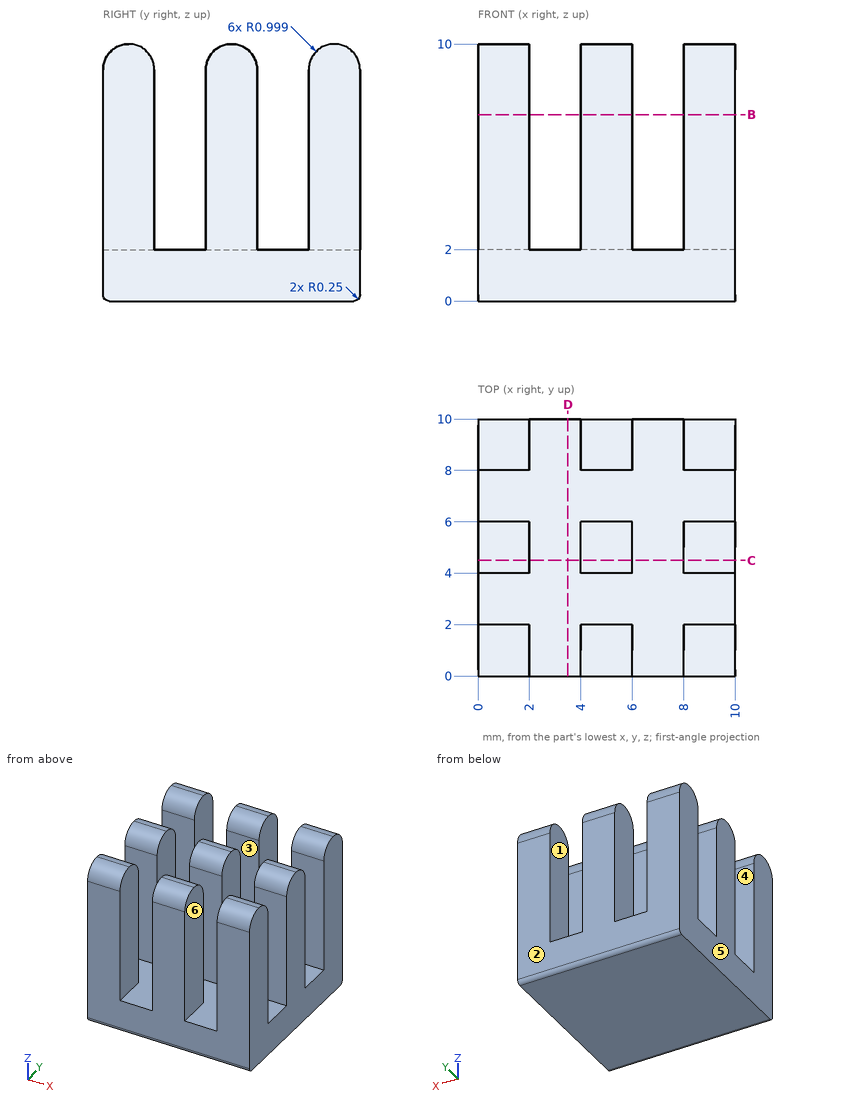
Job drawing, mm, ordinate dimensions from the low corner. One solid piece. A direction names the side the tool comes from. Give positions to 0.01 mm unless a question says otherwise; leave off trailing zeros. Write each loop counter-clockwise with the first axis right and the second up, starting at its lowest first coordinate (ties: lowest second). Pieces come first, ordered by that corner, then holes. Notation, with made-up numbers: (52.25, -23) - (107.25, -23) arc R14 ccw to (107.25, -12) - close; hole circle Ø11 at (9, 12). An arc over 180 degrees is marked (long way). Use one line per item in the form item = value. Start each with the question number.
1. Band-saw the part on D-D on x = 3.5. Write the cut outline in (y, z), plus the area to 3 significant figures.
2. Drop a flat-ended pin along its axis: pin 1 Ø2 at (x, y) = (5.5, 6.5) entering from +Z. Give the stop position or say it passes through.
3. Two-plate mould, pull along Y, no slides. Class the marked faces 1, 2 and 3: released by +Y, released by -Y, zero draft, split by the parting line, or undercut.
4. Band-saw the part on C-C on y = 4.5. Write the cut outline in (x, z).
5. Band-saw the part on B-B on z = 7.25. Count the separate pieces of the cut face and the enclosed holes in it, plus the area to 3 significant figures.
6. Probe line 1 (Y direction, x = 9.5, z = 8); line 2 (Z direction, x = 7.25, y = 4.25). List the from-to ranges inside material, lowest first. Write a range as [from, to].
7. 3-axis set-ups, long thin cutter, end or side, ignore diameter. For the marked faces 4, 5 and 6: which of +Z, -Z, +X, -X, +Y, -Y reach the whole face in a straight line?
Conclusion:
q1.outline = (0, 0.25) arc R0.25 ccw to (0.25, 0) - (9.75, 0) arc R0.25 ccw to (10, 0.25) - (10, 2) - (0, 2) - close
q1.area = 20.0 mm²
q2.pin_1 = 9.87
q3.face_1 = zero draft
q3.face_2 = released by +Y
q3.face_3 = undercut
q4.outline = (0, 0) - (10, 0) - (10, 9.87) - (8, 9.87) - (8, 2) - (6, 2) - (6, 9.87) - (4, 9.87) - (4, 2) - (2, 2) - (2, 9.87) - (0, 9.87) - close
q5.separate_pieces = 9
q5.enclosed_holes = 0
q5.area = 36.0 mm²
q6.line_1 = [0, 2], [4, 6], [8, 10]
q6.line_2 = [0, 2]
q7.face_4 = +Z, +X, -X
q7.face_5 = +Z, -Z, -X, +Y, -Y
q7.face_6 = +Z, +Y, -Y
